from build123d import *

# Parameters (mm, degrees)
F0_W        = 88
F0_H        = 42
F0_W_2      = 72
F0_H_2      = 27
F1_DEPTH    = 8.5
F3_DEPTH    = 4
F2_W        = 2.75
F2_H        = 5.9
F4_DEPTH    = 3.4
F5_T1_DEPTH = 93
F5_T3_DEPTH = 47


# Not quite as in the source:
# - a fillet or chamfer that OpenCascade refuses, or shapes differently, is made with other operations: its cross-section is extruded or revolved along the edge and cut away or added


with BuildPart() as f1:
    # F0 (on Top) → F1 (new body)
    with BuildSketch(Plane.XY):
        Rectangle(F0_W, F0_H)
        Rectangle(F0_W_2, F0_H_2, mode=Mode.SUBTRACT)
    extrude(amount=F1_DEPTH)

    # F2 (on face) → F3 (cut)
    with BuildSketch(Plane(origin=(0, 0, 0), x_dir=(1, 0, 0), z_dir=(0, 0, -1))):
        Polygon((38.75, 8.2), (36, 8.2), (36, -8.5), (38.75, -8.5), (38.75, -2.8), (38.75, 3.1), align=None)
    extrude(amount=-F3_DEPTH, mode=Mode.SUBTRACT)

    # F2 (on face) → F4 (cut)
    with BuildSketch(Plane(origin=(0, 0, 0), x_dir=(1, 0, 0), z_dir=(0, 0, -1))):
        Polygon((36, -8.5), (36, 8.2), (38.75, 8.2), (38.75, 3.1), (41.5, 3.1), (41.5, 18.1), (-39, 18.1), (-39, -18.2), (41.5, -18.2), (41.5, -2.8), (38.75, -2.8), (38.75, -8.5), align=None)
        with Locations((40.125, 0.15)):
            Rectangle(F2_W, F2_H)
    extrude(amount=-F4_DEPTH, mode=Mode.SUBTRACT)

    # F5: fillet of radius 1 on 4 edges, made by hand

    # F5_s2 → F5_t1 (cut)
    with BuildSketch(Plane.YZ.offset(-46.5)):
        with BuildLine():
            add(Edge.make_bspline(
                [(-20, 8.5), (-21, 8.5), (-21, 7.5)],
                knots=[0, 0, 0, 1, 1, 1], degree=2, weights=[1, 1, 1]))
            Line((-21, 7.5), (-21, 8.5))
            Line((-21, 8.5), (-20, 8.5))
        make_face()
        with BuildLine():
            add(Edge.make_bspline(
                [(21, 7.5), (21, 8.5), (20, 8.5)],
                knots=[0, 0, 0, 1, 1, 1], degree=2, weights=[1, 1, 1]))
            Line((20, 8.5), (21, 8.5))
            Line((21, 8.5), (21, 7.5))
        make_face()
    extrude(amount=F5_T1_DEPTH, mode=Mode.SUBTRACT)

    # F5_s4 → F5_t3 (cut)
    with BuildSketch(Plane.XZ.offset(-23.5)):
        with BuildLine():
            add(Edge.make_bspline(
                [(44, 7.5), (44, 8.5), (43, 8.5)],
                knots=[0, 0, 0, 1, 1, 1], degree=2, weights=[1, 1, 1]))
            Line((43, 8.5), (44, 8.5))
            Line((44, 8.5), (44, 7.5))
        make_face()
        with BuildLine():
            add(Edge.make_bspline(
                [(-44, 7.5), (-44, 8.5), (-43, 8.5)],
                knots=[0, 0, 0, 1, 1, 1], degree=2, weights=[1, 1, 1]))
            Line((-43, 8.5), (-44, 8.5))
            Line((-44, 8.5), (-44, 7.5))
        make_face()
    extrude(amount=F5_T3_DEPTH, mode=Mode.SUBTRACT)


solid = f1.part
Design review of the part built by this model. Coordinates are the model's own, in mm. A direction names the side the tool comes from. Round coordinates to 2 decimals unless told otherwise and drop trailing zeros. Order: outer loops, then holes, each group sorted by start corner. A loop starts at its lowest first (then second) coordinate and runs counter-clockwise, first axis right, second up. Notation, with made-up numbers: M 23.25,30 L 47.25,30 A24 cw 47.25,43 Z; hole C -18.5,47.25 d2. An arc over 180 degrees is marked long. Answer as CSV lines item,"result". Start each with the question number.
1) For pin 1 Ø3 at (x, y) = (37, -1) entering from -Z; pin 2 Ø5 at (x, y) = (-20, 13.5) entering from -Z, all flat-tipped, find the tip position at first contact; note any pin that passes through.
2) Tool access review of faces 4 (the face through (-44, 0, 4)), 5 (the face through (1, 15, 3.4)), 6 (the face through (36, 0, 6)): name each direction out of +Z, -Z, +X, -X, +Y, -Y from which nothing blocks a thin tool from reaching the whole face with its end or side.
3) Wall thickness on line 1 along Y through (x, z) = (20, 7.75); line 2 along Y through (x, z) = (-24.5, 1.75); line 3 along X through (y, z) = (8, 6): over which ranges is each line inside the solid? List them lowest first. Write a range as [from, to].
4) Add section A-A (z = 6.5). Give the boundary of the cut face in (x, y), then the cut area to 3 significant figures.
5) Add section B-B (z = 2.5). Give the boundary of the cut face in (x, y), then the cut area to 3 significant figures.
6) The part is to be moulded in two halves that separate along Y. For faces 1 (the face through (-1, 21, 4)), 2 (the face through (-1, 13.5, 6)), 3 (the face through (-1, 14, 8.5)), say which applies: +Y half, -Y half, draft (parallel to the pull), parting line (faces both ways), or undercut.
Resolved:
1,pin 1,"z = 4"
1,pin 2,"z = 3.4"
2,face 4,"+Z, -Z, -X, +Y, -Y"
2,face 5,"-Z"
2,face 6,"+Z, -Z"
3,line 1,"[-20.98, -13.5], [13.5, 20.98]"
3,line 2,"[-21, -18.1], [18.2, 21]"
3,line 3,"[-44, -36], [36, 44]"
4,outline,"M -44,-21 L 44,-21 L 44,21 L -44,21 Z; hole M -36,-13.5 L 36,-13.5 L 36,13.5 L -36,13.5 Z"
4,area,"1,750 mm^2"
5,outline,"M -44,-21 L 44,-21 L 44,21 L -44,21 Z; hole M -39,-18.1 L 41.5,-18.1 L 41.5,18.2 L -39,18.2 Z"
5,area,"774 mm^2"
6,face 1,"+Y half"
6,face 2,"undercut"
6,face 3,"draft"
